For this review, take the finished solid that the model builds, in its own axes (mm). Face numbers are marked on the shaded views. A direction names the side the tool comes from. Coordinates: 2 decimals unless noted, no trailing zeros. Loops run counter-clockwise (first coordinate to the right, second up) from the corner with the lowest first, then second, coordinate; pieces in that order, holes last. Notation, with made-up numbers: (79, 46.25) -> (90, 46.25) arc R20 ccw to (90, 67.25) -> close; hole circle Ø7 at (54.25, -40). An arc over 180 degrees is marked (long way). Answer in a Markdown table with one row per item.
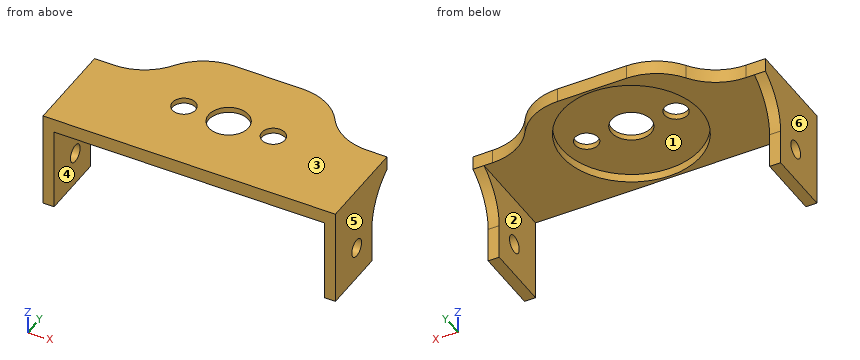
from build123d import *

# Parameters (mm, degrees)
BOSS_EXTRUDE1_DEPTH = 2.5
SKETCH4_R           = 12.55
CUT_EXTRUDE1_DEPTH  = 1.5
CUT_EXTRUDE2_REACH  = 33.444
SKETCH5_R           = 2.1
SKETCH5_R_2         = 3.6
SKETCH8_W           = 2
SKETCH8_H           = 12
BOSS_EXTRUDE3_DEPTH = 15
FILLET3_R           = 10
FILLET4_R           = 10
SKETCH9_R           = 1.6
CUT_EXTRUDE3_DEPTH  = 58.050444972


with BuildPart() as part:
    # Sketch3 → Boss-Extrude1 (new body)
    with BuildSketch(Plane.XY):
        Polygon((-11.828665208, 11.142231947), (14.171334792, 11.142231947), (14.171334792, 2.142231947), (27.671334792, 2.142231947), (27.671334792, -14.857768053), (-25.328665208, -14.857768053), (-25.328665208, 2.142231947), (-11.828665208, 2.142231947), align=None)
    extrude(amount=BOSS_EXTRUDE1_DEPTH)

    # Sketch4 → Cut-Extrude1 (cut)
    with BuildSketch(Plane(origin=(0, 0, 0), x_dir=(-1, 0, 0), z_dir=(0, 0, -1))):
        with Locations((-1.171334792, -1.857768053)):
            Circle(SKETCH4_R)
    extrude(amount=-CUT_EXTRUDE1_DEPTH, mode=Mode.SUBTRACT)

    # Sketch5 → Cut-Extrude2 (cut, up to next)
    with BuildSketch(Plane(origin=(0, 0, 1.5), x_dir=(-1, 0, 0), z_dir=(0, 0, -1)), mode=Mode.PRIVATE) as cut_extrude2_sk1:
        with Locations((-9.271334792, -1.857768053)):
            Circle(SKETCH5_R)
    cut_extrude2_tool1 = extrude(cut_extrude2_sk1.sketch, amount=-CUT_EXTRUDE2_REACH, mode=Mode.PRIVATE) & part.part
    # Sketch5 → Cut-Extrude2 (cut, up to next)
    with BuildSketch(Plane(origin=(0, 0, 1.5), x_dir=(-1, 0, 0), z_dir=(0, 0, -1)), mode=Mode.PRIVATE) as cut_extrude2_sk2:
        with Locations(Location((6.928665208, -1.857768053, 0), (0, 0, 180))):
            Circle(SKETCH5_R)
    cut_extrude2_tool2 = extrude(cut_extrude2_sk2.sketch, amount=-CUT_EXTRUDE2_REACH, mode=Mode.PRIVATE) & part.part
    # Sketch5 → Cut-Extrude2 (cut, up to next)
    with BuildSketch(Plane(origin=(0, 0, 1.5), x_dir=(-1, 0, 0), z_dir=(0, 0, -1)), mode=Mode.PRIVATE) as cut_extrude2_sk3:
        with Locations((-1.171334792, -1.857768053)):
            Circle(SKETCH5_R_2)
    cut_extrude2_tool3 = extrude(cut_extrude2_sk3.sketch, amount=-CUT_EXTRUDE2_REACH, mode=Mode.PRIVATE) & part.part
    add(cut_extrude2_tool1.solids().sort_by_distance((9.271335, -1.857768, 1.5))[0], mode=Mode.SUBTRACT)
    add(cut_extrude2_tool2.solids().sort_by_distance((-6.928665, -1.857768, 1.5))[0], mode=Mode.SUBTRACT)
    add(cut_extrude2_tool3.solids().sort_by_distance((1.171335, -1.857768, 1.5))[0], mode=Mode.SUBTRACT)

    # Sketch8 → Boss-Extrude3 (add)
    with BuildSketch(Plane(origin=(0, 0, 0), x_dir=(-1, 0, 0), z_dir=(0, 0, -1))):
        with Locations((-26.671334792, -8.857768053)):
            Rectangle(SKETCH8_W, SKETCH8_H)
        with Locations((24.328665208, -8.857768053)):
            Rectangle(SKETCH8_W, SKETCH8_H)
    extrude(amount=BOSS_EXTRUDE3_DEPTH)

    # Fillet3
    # the kernel refuses this fillet: 10 mm, written as the material it adds along each edge
    with BuildSketch(Plane(origin=(-11.828665208, 2.142231947, 0), x_dir=(-1, 0, 0), z_dir=(0, 0, 1))) as fillet3_piece_1:
        with BuildLine():
            CenterArc((9.949874371, -10), FILLET3_R, 90, 84.260829523)
            Line((0, -9), (-0.198997487, -8.98))
            ThreePointArc((-0.198997487, -8.98), (-0.2, -4.5), (-0.2, 0))
            Line((-0.2, 0), (0, 0.2))
            Line((0, 0.2), (9.949874371, 0.2))
            Line((9.949874371, 0.2), (9.949874371, 0))
        make_face()
    extrude(amount=2.5)
    with BuildSketch(Plane(origin=(14.171334792, 2.142231947, 0), x_dir=(1, 0, 0), z_dir=(0, 0, 1))) as fillet3_piece_2:
        with BuildLine():
            CenterArc((9.949874371, 10), FILLET3_R, 185.739170477, 84.260829523)
            Line((0, 9), (-0.198997487, 8.98))
            ThreePointArc((-0.198997487, 8.98), (-0.2, 4.5), (-0.2, 0))
            Line((-0.2, 0), (0, -0.2))
            Line((0, -0.2), (9.949874371, -0.2))
            Line((9.949874371, -0.2), (9.949874371, 0))
        make_face()
    extrude(amount=2.5)
    with BuildSketch(Plane(origin=(-23.328665208, -2.857768053, 0), x_dir=(0, 0, -1), z_dir=(-1, 0, 0)), Plane(origin=(27.671334792, -2.857768053, 0), x_dir=(0, 0, -1), z_dir=(-1, 0, 0))) as fillet3_piece_3:
        with BuildLine():
            CenterArc((8.660254038, -10), FILLET3_R, 90, 60)
            Line((0, -5), (-0.173205081, -4.9))
            ThreePointArc((-0.173205081, -4.9), (-0.2, -2.5), (-0.2, 0))
            Line((-0.2, 0), (0, 0.2))
            Line((0, 0.2), (8.660254038, 0.2))
            Line((8.660254038, 0.2), (8.660254038, 0))
        make_face()
    extrude(amount=2)

    # Fillet4
    fillet4_edges = [part.edges().sort_by_distance(p)[0] for p in [
        (-11.828665208, 11.142231947, 1.25),
        (14.171334792, 11.142231947, 1.25),
    ]]
    fillet(fillet4_edges, radius=FILLET4_R)

    # Sketch9 → Cut-Extrude3 (cut, through all)
    with BuildSketch(Plane(origin=(27.671334792, 0, 0), x_dir=(0, 0, -1), z_dir=(1, 0, 0))):
        with Locations((9, -7.857768053)):
            Circle(SKETCH9_R)
    extrude(amount=-CUT_EXTRUDE3_DEPTH, mode=Mode.SUBTRACT)


solid = part.part
Item 1: Take a section at B-B, the plane x = 8.5. State the section outline as (y, z) points, and give its area (3 significant figures).
Worked answers:
| item | result |
|---|---|
| outline | (-14.86, 0) -> (-12.05, 0) -> (-12.05, 1.5) -> (-3.81, 1.5) -> (-3.81, 2.5) -> (-14.86, 2.5) -> close; (0.1, 1.5) -> (8.33, 1.5) -> (8.33, 0) -> (11.08, 0) -> (11.08, 2.5) -> (0.1, 2.5) -> close |
| area | 30.4 mm² |
Item 2: Insertion check: pin 1 (8 mm diameter, centred on y = 7, z = 0.5, fed in from +X); pin 2 (0.8 mm diameter, centred on x = 26, z = 1, fed in from +Y); pin 3 (4.5 mm diameter, centred on y = -7.5, z = -10.5, fed in from -X); pin 4 (2 mm diameter, centred on x = -24.5, z = -10.5, fed in from +Y). Each pin has a flat end and moves straight along its axis. Give the tip position at first contact, or say it passes through.
Worked answers:
| item | result |
|---|---|
| pin 1 | x = 20.07 |
| pin 2 | y = 2.14 |
| pin 3 | x = -25.33 |
| pin 4 | y = -2.86 |
Item 3: Take a section at A-A, the plane z = -13. State the section outline as (x, y) points, and give its area (3 significant figures).
Worked answers:
| item | result |
|---|---|
| outline | (-25.33, -14.86) -> (-23.33, -14.86) -> (-23.33, -2.86) -> (-25.33, -2.86) -> close; (25.67, -14.86) -> (27.67, -14.86) -> (27.67, -2.86) -> (25.67, -2.86) -> close |
| area | 48.0 mm² |
Item 4: Take a section at D-D, the plane z = -5.25. State the section outline as (x, y) points, and give its area (3 significant figures).
Worked answers:
| item | result |
|---|---|
| outline | (-25.33, -14.86) -> (-23.33, -14.86) -> (-23.33, -2.26) -> (-25.33, -2.26) -> close; (25.67, -14.86) -> (27.67, -14.86) -> (27.67, -2.26) -> (25.67, -2.26) -> close |
| area | 50.4 mm² |
Item 5: Take a section at C-C, the plane y = 7.25. State the section outline as (x, z) points.
Worked answers:
| item | result |
|---|---|
| outline | (-12.99, 0) -> (-7.46, 0) -> (-7.46, 1.5) -> (9.81, 1.5) -> (9.81, 0) -> (15.34, 0) -> (15.34, 2.5) -> (-12.99, 2.5) -> close |
Item 6: For the marked faces 1, 2 and 3, list the 3-axis set-ups (+Z, -Z, +X, -X, +Y, -Y) from which the entire face can be reached by the end or side of a thin tool; tool diameter is ignored.
Worked answers:
| item | result |
|---|---|
| face 1 | -Z |
| face 2 | -Z, +Y, -Y |
| face 3 | +Z, +X, -X, +Y, -Y |
Item 7: For L1, parallel to X at y = -0.75, z = -0.25; L2, parallel to Z at x = -5.5, y = 6.75; L3, parallel to Z at x = -17, y = -13, list the stretches that pass through material, from the lowest coordinate up.
Worked answers:
| item | result |
|---|---|
| L1 | -25.33 to -23.33, 25.67 to 27.67 |
| L2 | 1.5 to 2.5 |
| L3 | 0 to 2.5 |
Item 8: The part is to be moulded in two halves that separate along X. For the marked faces 4, 5 and 6, say which applies: +X half, -X half, draft (parallel to the pull), parting line (faces both ways), or undercut.
Worked answers:
| item | result |
|---|---|
| face 4 | undercut |
| face 5 | +X half |
| face 6 | -X half |
